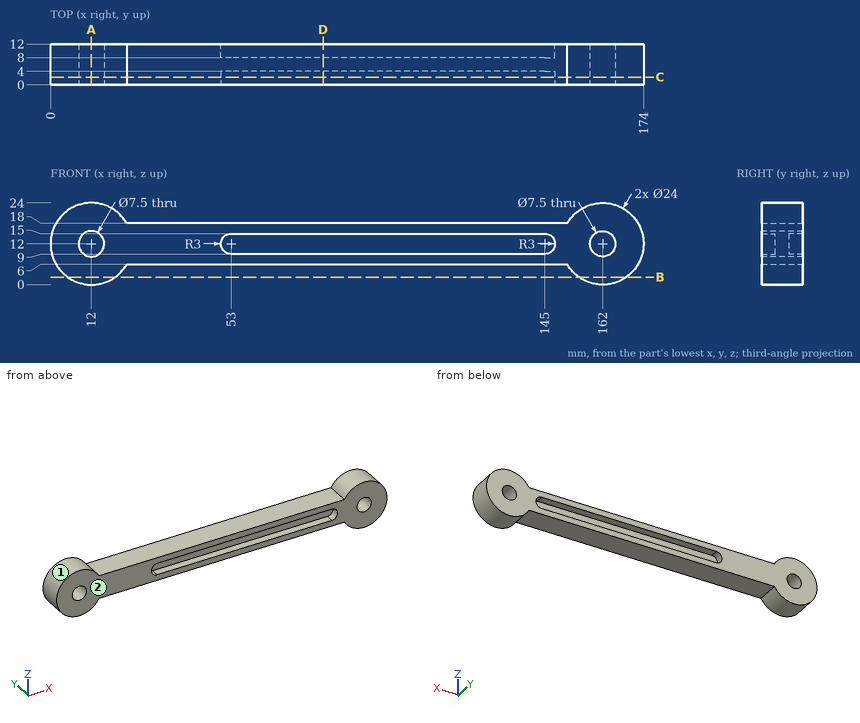
Part print with two shaded views. Sizes in mm from the minimum x, y, z corner. Coordinates: 2 decimals unless noted, no trailing zeros. Order: outer loops, then holes, each group sorted by start corner. A loop starts at its lowest first (then second) coordinate and runs counter-clockwise, first axis right, second up. Notation, with made-up numbers: M -16.5,-19.75 L -2.5,-19.75 A15 ccw -2.5,-5.75 Z; hole C 33,51.5 d3. An arc over 180 degrees is marked long. Use a Markdown table: item, result.
(1) Cut at D-D on x = 80. Write the cut outline in (y, z).
A:
| item | result |
|---|---|
| outline | M 0,6 L 12,6 L 12,9 L 8,9 L 8,15 L 12,15 L 12,18 L 0,18 L 0,15 L 4,15 L 4,9 L 0,9 Z |
(2) Pull direction X, two halves, no side cores. Call the marked faces 1 and 2: released by +X, released by -X, zero draft, split by the parting line, or undercut.
A:
| item | result |
|---|---|
| face 1 | undercut |
| face 2 | zero draft |
(3) Cut at B-B on z = 2.25. Write the cut outline in (x, y).
A:
| item | result |
|---|---|
| outline | M 5,0 L 19,0 L 19,12 L 5,12 Z; M 155,0 L 169,0 L 169,12 L 155,12 Z |
(4) Probe L1, parallel to Z at x = 72, y = 10; L2, parallel to X at y = 5.75, z = 12.25; L3, parallel to X at y = 5.5, z = 9. List the from-to ranges inside material, lowest first.
A:
| item | result |
|---|---|
| L1 | z = 6 to 9, 15 to 18 |
| L2 | x = 0 to 8.26, 15.74 to 158.26, 165.74 to 174 |
| L3 | x = 0.38 to 9.75, 14.25 to 159.75, 164.25 to 173.62 |
(5) Cut at C-C on y = 2.25. Write the cut outline in (x, z).
A:
| item | result |
|---|---|
| outline | M 22.39,6 L 151.61,6 A12 ccw long 151.61,18 L 22.39,18 A12 ccw long Z; hole C 12,12 d7.5; hole M 53,9 L 145,9 A3 ccw 145,15 L 53,15 A3 ccw Z; hole C 162,12 d7.5 |
(6) Cut at A-A on x = 12. Write the cut outline in (y, z).
A:
| item | result |
|---|---|
| outline | M 0,0 L 12,0 L 12,8.25 L 0,8.25 Z; M 0,15.75 L 12,15.75 L 12,24 L 0,24 Z |
(7) Flat gauge pins, fed straight in: pin 1 (1.5 mm diameter, centred on y = 6, z = 9, fed in from +X); pin 2 (4.5 mm diameter, centred on x = 106.5, y = 10, fed in from -Z); pin 3 (6 mm diameter, centred on y = 7.5, z = 15.5, fed in from -X); pin 4 (7 mm diameter, centred on x = 12, z = 12, fed in from +Y). Where does each tip first touch, or does it go through?
A:
| item | result |
|---|---|
| pin 1 | stops at x = 173.79 |
| pin 2 | stops at z = 6 |
| pin 3 | stops at x = 0.01 |
| pin 4 | passes through |
